```python
from build123d import *

# Parameters (mm, degrees)
PAD_DEPTH       = 18
SKETCH001_R     = 2.5
POCKET_DEPTH    = 18.501
CHAMFER_SIZE    = 2
CHAMFER001_SIZE = 1.5


with BuildPart() as part:
    # Sketch → Pad (new body)
    with BuildSketch(Plane.XY):
        with BuildLine():
            Line((-6.145128, -9.214477), (16.854872, -9.214477))
            Line((16.854872, -9.214477), (16.854872, 2.985523))
            Line((11.963718, 2.985523), (16.854872, 2.985523))
            ThreePointArc((11.963718, 2.985523), (5.37466, 8.550501), (7.839372, 0.285523))
            Line((13.854872, 0.285523), (7.839372, 0.285523))
            Line((13.854872, -6.214477), (13.854872, 0.285523))
            Line((-6.145128, -6.214477), (13.854872, -6.214477))
            Line((-6.145128, -9.214477), (-6.145128, -6.214477))
        make_face()
    extrude(amount=PAD_DEPTH)

    # Sketch001 → Pocket (cut, through all)
    with BuildSketch(Plane.XZ.offset(9.214477)):
        with Locations((2.854872, 9)):
            Circle(SKETCH001_R)
    extrude(amount=-POCKET_DEPTH, mode=Mode.SUBTRACT)

    # Chamfer
    chamfer_edges = [part.edges().sort_by_distance(p)[0] for p in [
        (0.354872, -6.214477, 9),
    ]]
    chamfer(chamfer_edges, length=CHAMFER_SIZE)

    # Chamfer001
    chamfer001_edges = [part.edges().sort_by_distance(p)[0] for p in [
        (11.963718, 2.985523, 9),
    ]]
    chamfer(chamfer001_edges, length=CHAMFER001_SIZE)


solid = part.part
```
Input: part model. Units: mm. Frame: model coordinates. A direction names the side the tool comes from. Give positions to 0.01 mm unless a question says otherwise; leave off trailing zeros. Order: outer loops, then holes, each group sorted by start corner. A loop starts at its lowest first (then second) coordinate and runs counter-clockwise, first axis right, second up. Notation, with made-up numbers: M -19.5,89.25 L -6.5,89.25 A5 ccw -6.5,95.25 Z; hole C -29,2 d6. An arc over 180 degrees is marked long. Return JSON: item names as keys, results as strings.
Item 1: Cut plane B-B (y = -7). Return loops of the section in (x, z).
Solutions:
{"outline": "M -6.15,0 L 16.85,0 L 16.85,18 L -6.15,18 Z; hole C 2.85,9 d7.43"}
Item 2: Cut plane D-D (y = 6.75). Return loops of the section in (x, z).
Solutions:
{"outline": "M 3.79,0 L 11.89,0 L 11.89,18 L 3.79,18 L 3.79,11.32 A2.5 cw 3.79,6.68 Z"}
Item 3: Cut plane A-A (z = 9). Return loops of the section in (x, y).
Solutions:
{"outline": "M -6.15,-9.21 L 0.35,-9.21 L 0.35,-8.21 L -1.65,-6.21 L -6.15,-6.21 Z; M 5.35,-9.21 L 16.85,-9.21 L 16.85,2.99 L 13.46,2.99 L 12.33,4.44 A4.5 ccw 5.35,8.54 L 5.35,1.03 A4.5 ccw 7.84,0.29 L 13.85,0.29 L 13.85,-6.21 L 7.35,-6.21 L 5.35,-8.21 Z"}
Item 4: Pull-direction query (X, two-part tool) for faces 1 (the flat face through (-6.145, -8, 9)), 2 (the conical face through (2.286, -8.089, 6.437)), 3 (the flat face through (8, 1, 0)); classes: +X half, -X half, draft (parallel to the pull), parting line (faces both ways), or undercut.
Solutions:
{"face 1": "-X half", "face 2": "undercut", "face 3": "draft"}
Item 5: Cut plane C-C (x = 4.25). State how many separate pieces and enclosed holes the cut face has, then the cut area to 3 significant figures.
Solutions:
{"separate pieces": "4", "enclosed holes": "0", "area": "112 mm^2"}
Item 6: Access query for faces 4 (the flat face through (15, 2.986, 9)), 5 (the flat face through (8, -6.214, 9)), 6 (the cylindrical face through (5.354, 4.733, 8.952)). Directions: +Z, -Z, +X, -X, +Y, -Y. A direction counts if a zero-diameter tool reaches every point of the face in a straight line with its end or side. Return the directions, or none.
Solutions:
{"face 4": "+Z, -Z, +X, +Y", "face 5": "+Z, -Z, -X", "face 6": "-X, +Y, -Y"}
Item 7: Ray query, probe 1 along Y at (x, z) = (13.75, 16.75); probe 2 along Y at (x, z) = (0, 1.5); probe 3 along X at (y, z) = (-0.25, 11.5). Return the intervals inside material, ascending.
Solutions:
{"probe 1": "-9.21 to -6.21, 0.29 to 2.99", "probe 2": "-9.21 to -6.21", "probe 3": "13.85 to 16.85"}
Item 8: First-contact query: P1, Ø2.5, axis at x = 14.5, z = 6.5, coming from the +Y side; P2, Ø4.5, axis at x = 2.85, z = 9, coming from the -Y side; P3, Ø9, axis at x = 8.5, z = 12, coming from the +Y side; P4, Ø3, axis at y = -4.5, z = 9, coming from the -X side. Flat tips, straight axial feed; report the tip coordinate or a pass-through.
Solutions:
{"P1": "y = 3.26", "P2": "through", "P3": "y = 9.29", "P4": "x = 13.85"}
